from build123d import *

# Parameters (mm, degrees)
SKETCH_1_R           = 14
EXTRUDE_1_DEPTH      = 22
SKETCH_3_R           = 7.35
CUT_EXTRUDE_1_DEPTH  = 6
SKETCH_2_R           = 1.1
CUT_EXTRUDE_2_DEPTH  = 32
SKETCH_4_R           = 1.9
SKETCH_4_R_2         = 1.85
CUT_EXTRUDE_3_DEPTH  = 19
SKETCH_5_W           = 5.15
SKETCH_5_H           = 5.15
CUT_EXTRUDE_4_DEPTH  = 13
EXTRUDE_2_REACH      = 32.899
SKETCH_12_R          = 19.208398283
CUT_EXTRUDE_9_DEPTH  = 4
FILLET_1_R           = 2
SKETCH_14_R          = 2.5
CUT_EXTRUDE_10_DEPTH = 18
SKETCH_15_R          = 4.075
CUT_EXTRUDE_11_DEPTH = 2


with BuildPart() as part:
    # 草图1 → 凸台-拉伸1 (new body)
    with BuildSketch(Plane.XY):
        Circle(SKETCH_1_R)
    extrude(amount=EXTRUDE_1_DEPTH)

    # 草图3 → 切除-拉伸1 (cut)
    with BuildSketch(Plane(origin=(0, 0, 0), x_dir=(-1, 0, 0), z_dir=(0, 0, -1))):
        Circle(SKETCH_3_R)
    extrude(amount=-CUT_EXTRUDE_1_DEPTH, mode=Mode.SUBTRACT)

    # 草图2 → 切除-拉伸2 (cut)
    with BuildSketch(Plane.XY.offset(22)):
        with Locations((-9.09326674, 5.25)):
            Circle(SKETCH_2_R)
        with Locations((9.09326674, 5.25)):
            Circle(SKETCH_2_R)
        with Locations((0, -10.5)):
            Circle(SKETCH_2_R)
    extrude(amount=-CUT_EXTRUDE_2_DEPTH, mode=Mode.SUBTRACT)

    # 草图4 → 切除-拉伸3 (cut)
    with BuildSketch(Plane.XY.offset(22)):
        with Locations((9.09326674, 5.25)):
            Circle(SKETCH_4_R)
        with Locations((0, -10.5)):
            Circle(SKETCH_4_R)
        with Locations((-9.09326674, 5.25)):
            Circle(SKETCH_4_R_2)
    extrude(amount=-CUT_EXTRUDE_3_DEPTH, mode=Mode.SUBTRACT)

    # 草图5 → 切除-拉伸4 (cut)
    with BuildSketch(Plane.XY.offset(22)):
        Rectangle(SKETCH_5_W, SKETCH_5_H)
    extrude(amount=-CUT_EXTRUDE_4_DEPTH, mode=Mode.SUBTRACT)

    # 草图6 → 凸台-拉伸2 (add, up to next)
    with BuildSketch(Plane(origin=(-2.575, 0, 0), x_dir=(0, 0, -1), z_dir=(1, 0, 0)), mode=Mode.PRIVATE) as extrude_2_sk1:
        Polygon((-9, -2.575), (-14.15, -2.575), (-9, 2.575), align=None)
    extrude_2_tool1 = extrude(extrude_2_sk1.sketch, amount=EXTRUDE_2_REACH, mode=Mode.PRIVATE) - part.part
    add(extrude_2_tool1.solids().sort_by_distance((-2.575, -0.858333, 10.716667))[0])

    # 草图12 → 切除-拉伸9 (cut)
    with BuildSketch(Plane.XY.offset(22)):
        Circle(SKETCH_12_R)
    extrude(amount=-CUT_EXTRUDE_9_DEPTH, mode=Mode.SUBTRACT)

    # 圆角1
    # the kernel refuses this fillet: 2 mm, written as the material it takes off along each edge
    with BuildSketch(Plane(origin=(0, 0, 18), x_dir=(1, 0, 0), z_dir=(0, 1, 0))) as fillet_1_piece_1:
        with BuildLine():
            CenterArc((14 - FILLET_1_R, FILLET_1_R), FILLET_1_R, 270, 90)
            Line((14, FILLET_1_R), (14, 0))
            Line((14, 0), (14 - FILLET_1_R, 0))
        make_face()
    revolve(axis=Axis((0, 0, 18), (0, 0, -1)), mode=Mode.SUBTRACT)

    # 草图14 → 切除-拉伸10 (cut)
    with BuildSketch(Plane(origin=(0, 2.575, 0), x_dir=(-1, 0, 0), z_dir=(0, -1, 0))):
        with Locations(Location((0, -11.575, 0), (0, 0, 90))):
            Circle(SKETCH_14_R)
    extrude(amount=-CUT_EXTRUDE_10_DEPTH, mode=Mode.SUBTRACT)

    # 草图15 → 切除-拉伸11 (cut, symmetric)
    with BuildSketch(Plane(origin=(0, 13.416407865, 0), x_dir=(1, 0, 0), z_dir=(0, 1, 0))):
        with Locations(Location((0, -11.575, 0), (0, 0, 270))):
            Circle(SKETCH_15_R)
    extrude(amount=CUT_EXTRUDE_11_DEPTH, both=True, mode=Mode.SUBTRACT)


solid = part.part
Part model, mm, in its own coordinate system. A direction names the side the tool comes from. Give positions to 0.01 mm unless a question says otherwise; leave off trailing zeros. Order: outer loops, then holes, each group sorted by start corner. A loop starts at its lowest first (then second) coordinate and runs counter-clockwise, first axis right, second up. Notation, with made-up numbers: (55.5, -6) - (109.5, -6) arc R12 ccw to (109.5, 7) - close; hole circle Ø1 at (72, 49.25). An arc over 180 degrees is marked (long way). Use a Markdown table: item, result.
1) Flat gauge pins, fed straight in: P1, Ø2.5, axis at x = -2, z = 11.5, coming from the +Y side; P2, Ø2, axis at x = 0, y = -10.5, coming from the +Z side; P3, Ø1.5, axis at y = 6, z = 6.5, coming from the +X side; P4, Ø1.5, axis at x = -9.5, z = 5, coming from the -Y side. Where does each tip first touch, or does it go through?
Checked values:
| item | result |
|---|---|
| P1 | y = 11.42 |
| P2 | through |
| P3 | x = 12.98 |
| P4 | y = -10.93 |
2) Saw through at C-C on z = 11.5. List the corners of the cut face in (x, y) (3 decimals), plus the area to 3 significant figures.
Checked values:
| item | result |
|---|---|
| outline | (-4.074, 11.416) - (-4.074, 13.394) arc R14 ccw (long way) to (4.074, 13.394) - (4.074, 11.416) - (2.499, 11.416) - (2.499, 2.575) - (2.575, 2.575) - (2.575, 0.075) - (-2.575, 0.075) - (-2.575, 2.575) - (-2.499, 2.575) - (-2.499, 11.416) - close; hole circle Ø3.7 at (-9.093, 5.25); hole circle Ø3.8 at (0, -10.5); hole circle Ø3.8 at (9.093, 5.25) |
| area | 506 mm² |
3) Saw through at A-A on z = 15. List the corners of the cut face in (x, y) (3 decimals), plus the area to 3 significant figures.
Checked values:
| item | result |
|---|---|
| outline | (-2.208, 11.416) - (-2.208, 13.825) arc R14 ccw (long way) to (2.208, 13.825) - (2.208, 11.416) - close; hole circle Ø3.7 at (-9.093, 5.25); hole (-2.575, -2.575) - (2.575, -2.575) - (2.575, 2.575) - (-2.575, 2.575) - close; hole circle Ø3.8 at (0, -10.5); hole circle Ø3.8 at (9.093, 5.25) |
| area | 545 mm² |
4) Two-plate mould, pull along X, no slides. Class faces 1 (the cylindrical face through (-3.03, -13.67, 7.89)), 2 (the flat face through (-3, 0, 18)), 3 (the cylindrical face through (1.593, -7.175, 2.958)): +X half, -X half, draft (parallel to the pull), parting line (faces both ways), or undercut.
Checked values:
| item | result |
|---|---|
| face 1 | parting line |
| face 2 | draft |
| face 3 | undercut |
5) Probe L1, parallel to Z at x = -0.5, y = 5.25; L2, parallel to Z at x = 4.25, y = -4.5; L3, parallel to X at y = 3.25, z = 11.5. List the from-to ranges inside material, lowest first. Write a range as from..to.
Checked values:
| item | result |
|---|---|
| L1 | 6..9.13, 14.02..18 |
| L2 | 6..18 |
| L3 | -13.62..-2.5, 2.5..13.62 |
6) Saw through at B-B on x = 0. Count the separate pieces of the cut face and the enclosed holes in it, plus the area to 3 significant figures.
Checked values:
| item | result |
|---|---|
| separate pieces | 3 |
| enclosed holes | 0 |
| area | 252 mm² |
7) Saw through at D-D on y = 0. List the corners of the cut face in (x, z) (3 decimals).
Checked values:
| item | result |
|---|---|
| outline | (-14, 0) - (-7.35, 0) - (-7.35, 6) - (7.35, 6) - (7.35, 0) - (14, 0) - (14, 16) arc R2 ccw to (12, 18) - (2.575, 18) - (2.575, 11.575) - (-2.575, 11.575) - (-2.575, 18) - (-12, 18) arc R2 ccw to (-14, 16) - close |
8) 3-axis set-ups, long thin cutter, end or side, ignore diameter. For faces 4 (the flat face through (0, 0, 6)), 5 (the flat face through (0.06, 11.416, 14.23)), 6 (the flat face through (-2.575, 1, 15)): which of +Z, -Z, +X, -X, +Y, -Y reach the whole face in a straight line?
Checked values:
| item | result |
|---|---|
| face 4 | -Z |
| face 5 | +Y |
| face 6 | +Z |
